Geometry: see drawing. Coordinates: mm, zero at the bounding-box minimum. Coordinates: 2 decimals unless noted, no trailing zeros. Order: outer loops, then holes, each group sorted by start corner. A loop starts at its lowest first (then second) coordinate and runs counter-clockwise, first axis right, second up. Notation, with made-up numbers: M 35.5,-17 L 46.5,-17 A30 ccw 46.5,18 Z; hole C 39,-1 d3. An arc over 180 degrees is marked long. One line per item, written item: value.
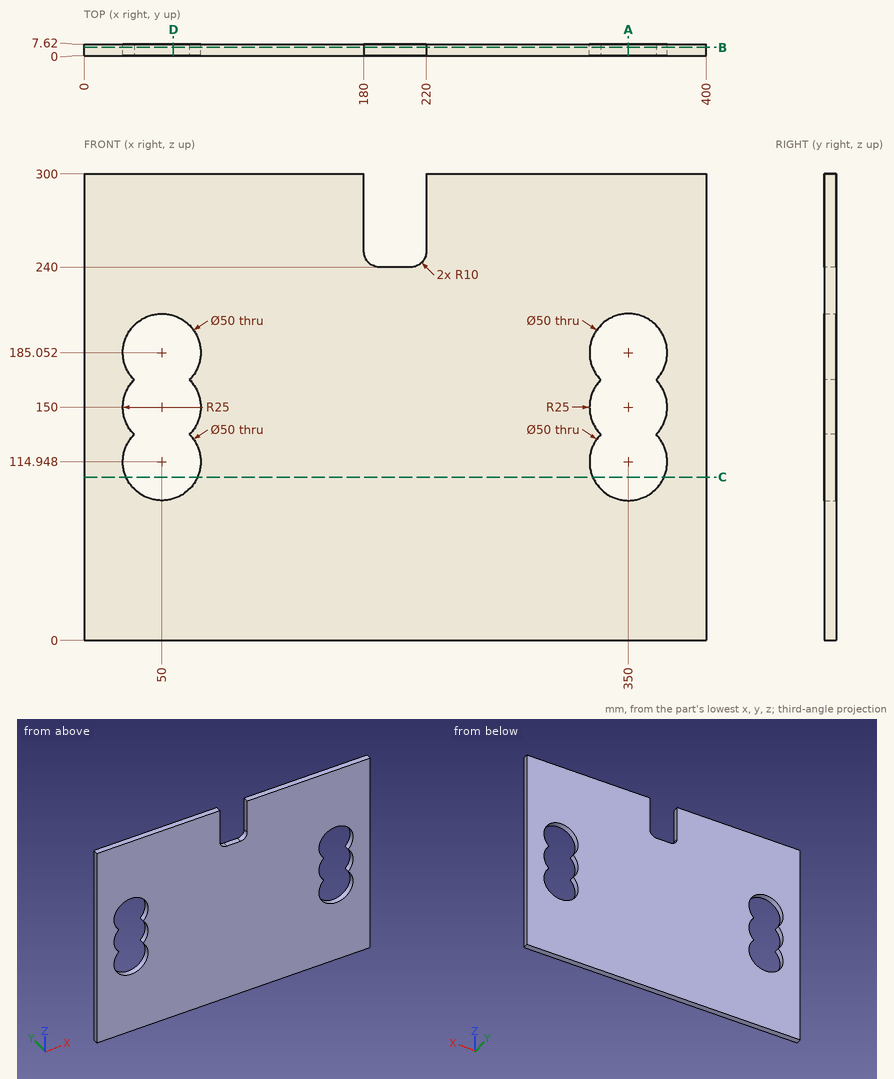
(1) Cut plane A-A on x = 350. Output: boundary loops of the cut face in (y, z).
Data:
outline: M 0,0 L 7.62,0 L 7.62,89.95 L 0,89.95 Z; M 0,210.05 L 7.62,210.05 L 7.62,300 L 0,300 Z
(2) Cut plane D-D on x = 57.5. Output: boundary loops of the cut face in (y, z), plus the area to 3 significant figures.
Data:
outline: M 0,0 L 7.62,0 L 7.62,91.1 L 0,91.1 Z; M 0,208.9 L 7.62,208.9 L 7.62,300 L 0,300 Z
area: 1,390 mm2
(3) Cut plane C-C on z = 105. Output: boundary loops of the cut face in (x, y), plus the area to 3 significant figures.
Data:
outline: M 0,0 L 27.06,0 L 27.06,7.62 L 0,7.62 Z; M 72.94,0 L 327.06,0 L 327.06,7.62 L 72.94,7.62 Z; M 372.94,0 L 400,0 L 400,7.62 L 372.94,7.62 Z
area: 2,350 mm2
(4) Ray query, line 1 (Z direction, x = 50, y = 4); line 2 (X direction, y = 2.5, z = 132); line 3 (X direction, y = 2.5, z = 287). Return the intervals inside material, ascending. Write a range as from..to.
Data:
line 1: z = 0..89.95, 210.05..300
line 2: x = 0..31.72, 68.28..331.72, 368.28..400
line 3: x = 0..180, 220..400
(5) Cut plane B-B on y = 5.5. Output: boundary loops of the cut face in (x, z), plus the area to 3 significant figures.
Data:
outline: M 0,0 L 400,0 L 400,300 L 220,300 L 220,250 A10 cw 210,240 L 190,240 A10 cw 180,250 L 180,300 L 0,300 Z; hole M 32.17,132.47 A25 ccw long 67.83,132.47 A25 ccw 67.83,167.53 A25 ccw long 32.17,167.53 A25 ccw Z; hole M 332.17,132.47 A25 ccw long 367.83,132.47 A25 ccw 367.83,167.53 A25 ccw long 332.17,167.53 A25 ccw Z
area: 107,000 mm2
(6) First-contact query: pin 1 (2.5 mm diameter, centred on x = 197.5, y = 4.5, fed in from +Z). Flat tip, straight axial feed; report the tip coordinate or a pass-through.
Data:
pin 1: stops at z = 240
